For this review, take the finished solid that the model builds, in its own axes (mm). Give positions to 0.01 mm unless a question says otherwise; leave off trailing zeros. Order: outer loops, then holes, each group sorted by start corner. A loop starts at its lowest first (then second) coordinate and runs counter-clockwise, first axis right, second up. Notation, with made-up numbers: (-21, 31.25) - (4, 31.25) arc R19 cw to (4, 62.25) - close; hole circle Ø6 at (-15, -31). An arc over 180 degrees is marked (long way). Use a Markdown table: item, result. Add a question column.
1) Mouldability with a two-part tool opening along X and no side actions: class faces 1 (the face through (100, 2, -49)), 2 (the face through (0, 2, -49)), 3 (the face through (9.102, 2.465, -51.474)), 4 (the face through (49, 0, -51)) as released by +X, released by -X, zero draft, split by the parting line, or undercut.
2) We need section B-B on z = -70. Write out the cut boundary in (x, y).
3) Clearance check with a flat-ended pin moving along its axis: P1, Ø3, axis at x = 20.12, z = -20.12, coming from the +Y side. State where the tip first meets the part, or that it passes through.
4) We need section C-C on z = -92.25. Write out the cut boundary in (x, y), then the cut area to 3 significant figures.
5) We need section A-A on x = 92.25. Write out the cut boundary in (y, z).
6) We need section D-D on z = -20. Write out the cut boundary in (x, y), then the cut area to 3 significant figures.
7) Wall thickness on L1, parallel to X at y = 2.9, z = -50; L2, parallel to Z at x = 6, y = 3.8; L3, parallel to X at y = 1.7, z = -81: over which ranges is each line inside the solid? List them lowest first.
```python
from build123d import *

# Parameters (mm, degrees)
SKETCH2_W           = 100
SKETCH2_H           = 100
SKETCH2_R           = 2
SKETCH2_R_2         = 1.75
BOSS_EXTRUDE1_DEPTH = 5


with BuildPart() as part:
    # Sketch2 → Boss-Extrude1 (new body)
    with BuildSketch(Plane(origin=(0, 0, 0), x_dir=(1, 0, 0), z_dir=(0, 1, 0))):
        with Locations((50, 50)):
            Rectangle(SKETCH2_W, SKETCH2_H)
        with Locations(Location((50, 92.25, 0), (0, 0, 270))):
            Circle(SKETCH2_R, mode=Mode.SUBTRACT)
        with Locations(Location((79.875261505, 79.875261505, 0), (0, 0, 270))):
            Circle(SKETCH2_R, mode=Mode.SUBTRACT)
        with Locations(Location((92.25, 50, 0), (0, 0, 270))):
            Circle(SKETCH2_R, mode=Mode.SUBTRACT)
        with Locations(Location((79.875261505, 20.124738495, 0), (0, 0, 270))):
            Circle(SKETCH2_R, mode=Mode.SUBTRACT)
        with Locations(Location((50, 7.75, 0), (0, 0, 270))):
            Circle(SKETCH2_R, mode=Mode.SUBTRACT)
        with Locations(Location((20.124738495, 20.124738495, 0), (0, 0, 270))):
            Circle(SKETCH2_R, mode=Mode.SUBTRACT)
        with Locations(Location((7.75, 50, 0), (0, 0, 270))):
            Circle(SKETCH2_R, mode=Mode.SUBTRACT)
        with Locations(Location((20.124738495, 79.875261505, 0), (0, 0, 270))):
            Circle(SKETCH2_R, mode=Mode.SUBTRACT)
        with Locations(Location((2.5, 20, 0), (0, 0, 270))):
            Circle(SKETCH2_R_2, mode=Mode.SUBTRACT)
        with Locations(Location((2.5, 70, 0), (0, 0, 90))):
            Circle(SKETCH2_R_2, mode=Mode.SUBTRACT)
        with Locations(Location((97.5, 20, 0), (0, 0, 90))):
            Circle(SKETCH2_R_2, mode=Mode.SUBTRACT)
        with Locations(Location((97.5, 70, 0), (0, 0, 270))):
            Circle(SKETCH2_R_2, mode=Mode.SUBTRACT)
    extrude(amount=BOSS_EXTRUDE1_DEPTH)


solid = part.part
```
Checked values:
| question | item | result |
|---|---|---|
| 1 | face 1 | released by +X |
| 1 | face 2 | released by -X |
| 1 | face 3 | undercut |
| 1 | face 4 | zero draft |
| 2 | outline | (0, 0) - (0.75, 0) - (0.75, 5) - (0, 5) - close; (4.25, 0) - (95.75, 0) - (95.75, 5) - (4.25, 5) - close; (99.25, 0) - (100, 0) - (100, 5) - (99.25, 5) - close |
| 3 | P1 | through |
| 4 | outline | (0, 0) - (48, 0) - (48, 5) - (0, 5) - close; (52, 0) - (100, 0) - (100, 5) - (52, 5) - close |
| 4 | area | 480 mm² |
| 5 | outline | (0, -100) - (5, -100) - (5, -52) - (0, -52) - close; (0, -48) - (5, -48) - (5, 0) - (0, 0) - close |
| 6 | outline | (0, 0) - (0.75, 0) - (0.75, 5) - (0, 5) - close; (4.25, 0) - (18.13, 0) - (18.13, 5) - (4.25, 5) - close; (22.12, 0) - (77.88, 0) - (77.88, 5) - (22.12, 5) - close; (81.87, 0) - (95.75, 0) - (95.75, 5) - (81.87, 5) - close; (99.25, 0) - (100, 0) - (100, 5) - (99.25, 5) - close |
| 6 | area | 425 mm² |
| 7 | L1 | 0 to 5.75, 9.75 to 90.25, 94.25 to 100 |
| 7 | L2 | -100 to -50.97, -49.03 to 0 |
| 7 | L3 | 0 to 18.47, 21.78 to 78.22, 81.53 to 100 |
